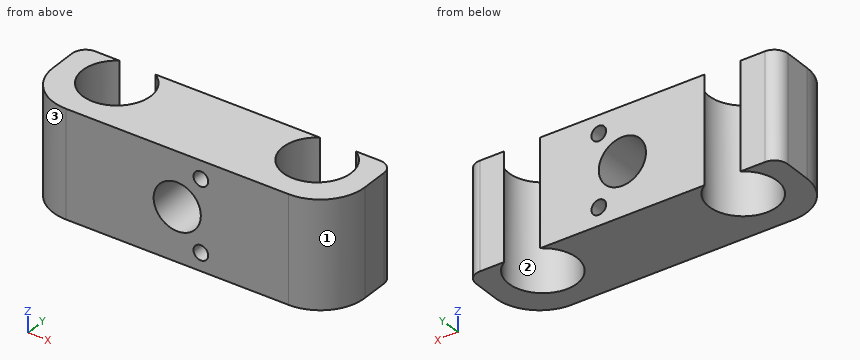
from build123d import *

# Parameters (mm, degrees)
SKETCH_1_W          = 70
SKETCH_1_H          = 19
EXTRUDE_1_DEPTH     = 24
SKETCH_2_R          = 7.65
CUT_EXTRUDE_1_DEPTH = 24
SKETCH_3_R          = 5.3
CUT_EXTRUDE_2_DEPTH = 24
FILLET_1_R          = 10
FILLET_4_R          = 3
FILLET_5_R          = 10
FILLET_6_R          = 3
SKETCH_4_R          = 1.65
CUT_EXTRUDE_3_DEPTH = 24


with BuildPart() as part:
    # 草图1 → 凸台-拉伸1 (new body)
    with BuildSketch(Plane.XY):
        with Locations((35, 9.5)):
            Rectangle(SKETCH_1_W, SKETCH_1_H)
    extrude(amount=EXTRUDE_1_DEPTH)

    # 草图2 → 切除-拉伸1 (cut)
    with BuildSketch(Plane.XY.offset(24)):
        with Locations((57.5, 12.5)):
            Circle(SKETCH_2_R)
        with Locations((12.5, 12.5)):
            Circle(SKETCH_2_R)
    extrude(amount=-CUT_EXTRUDE_1_DEPTH, mode=Mode.SUBTRACT)

    # 草图3 → 切除-拉伸2 (cut)
    with BuildSketch(Plane.XZ):
        with Locations((35, 12)):
            Circle(SKETCH_3_R)
    extrude(amount=-CUT_EXTRUDE_2_DEPTH, mode=Mode.SUBTRACT)

    # 圆角1
    fillet_1_edges = [part.edges().sort_by_distance(p)[0] for p in [
        (0, 0, 12),
    ]]
    fillet(fillet_1_edges, radius=FILLET_1_R)

    # 圆角4
    fillet_4_edges = [part.edges().sort_by_distance(p)[0] for p in [
        (0, 19, 12),
    ]]
    fillet(fillet_4_edges, radius=FILLET_4_R)

    # 圆角5
    fillet_5_edges = [part.edges().sort_by_distance(p)[0] for p in [
        (70, 0, 12),
    ]]
    fillet(fillet_5_edges, radius=FILLET_5_R)

    # 圆角6
    fillet_6_edges = [part.edges().sort_by_distance(p)[0] for p in [
        (70, 19, 12),
    ]]
    fillet(fillet_6_edges, radius=FILLET_6_R)

    # 草图4 → 切除-拉伸3 (cut)
    with BuildSketch(Plane(origin=(0, 19, 0), x_dir=(1, 0, 0), z_dir=(0, 1, 0))):
        with Locations((40.3, -20)):
            Circle(SKETCH_4_R)
        with Locations((40.3, -4)):
            Circle(SKETCH_4_R)
    extrude(amount=-CUT_EXTRUDE_3_DEPTH, mode=Mode.SUBTRACT)


solid = part.part
For this review, take the finished solid that the model builds, in its own axes (mm). Face numbers are marked on the shaded views. Round coordinates to 2 decimals unless told otherwise and drop trailing zeros. Loops run counter-clockwise (first coordinate to the right, second up) from the corner with the lowest first, then second, coordinate; pieces in that order, holes last. Notation, with made-up numbers: (9, 67.25) - (31, 67.25) arc R34 ccw to (31, 102.25) - close; hole circle Ø7 at (29, 5.5). An arc over 180 degrees is marked (long way). Put each result on its own line as item: value. Start each with the question number.
1. Consider section C-C on x = 35. State the section outline as (y, z) points, plus the area to 3 significant figures.
2. Consider section D-D on y = 8.5. State the section outline as (x, z) points, plus the area to 3 significant figures.
3. Consider section B-B on z = 4. State the section outline as (x, y) points, plus the area to 3 significant figures.
4. Mouldability with a two-part tool opening along X and no side actions: class the marked faces 1, 2 and 3 as +X half, -X half, draft (parallel to the pull), parting line (faces both ways), or undercut.
5. Insertion check: P1, Ø2.5, axis at x = 40.3, z = 20, coming from the +Y side; P2, Ø4, axis at y = 7, z = 15.5, coming from the -X side. Each pin has a flat end and moves straight along its axis. Give the tip position at first contact, or say it passes through.
6. Consider section A-A on y = 5.75. State the section outline as (x, z) points.
7. For probe 1 along X at (y, z) = (13.25, 4); probe 2 along X at (y, z) = (12.5, 12.5); probe 3 along Y at (x, z) = (12.5, 8.25), list the stretches that pass through material, from the lowest coordinate up. Write a range as [from, to].
Result sheet:
1. outline: (0, 0) - (19, 0) - (19, 6.7) - (0, 6.7) - close; (0, 17.3) - (19, 17.3) - (19, 24) - (0, 24) - close
1. area: 255 mm^2
2. outline: (0.11, 0) - (5.98, 0) - (5.98, 24) - (0.11, 24) - close; (19.02, 0) - (50.98, 0) - (50.98, 24) - (19.02, 24) - close; (64.02, 0) - (69.89, 0) - (69.89, 24) - (64.02, 24) - close; hole circle Ø10.6 at (35, 12); hole circle Ø3.3 at (40.3, 4); hole circle Ø3.3 at (40.3, 20)
2. area: 943 mm^2
3. outline: (0, 10) arc R10 ccw to (10, 0) - (38.65, 0) - (38.65, 19) - (16.53, 19) arc R7.65 cw (long way) to (8.47, 19) - (3, 19) arc R3 ccw to (0, 16) - close; (41.95, 0) - (60, 0) arc R10 ccw to (70, 10) - (70, 16) arc R3 ccw to (67, 19) - (61.53, 19) arc R7.65 cw (long way) to (53.47, 19) - (41.95, 19) - close
3. area: 865 mm^2
4. face 1: +X half
4. face 2: undercut
4. face 3: -X half
5. P1: through
5. P2: x = 0.05
6. outline: (0.95, 0) - (8.9, 0) - (8.9, 24) - (0.95, 24) - close; (16.1, 0) - (53.9, 0) - (53.9, 24) - (16.1, 24) - close; (61.1, 0) - (69.05, 0) - (69.05, 24) - (61.1, 24) - close; hole circle Ø10.6 at (35, 12); hole circle Ø3.3 at (40.3, 4); hole circle Ø3.3 at (40.3, 20)
7. probe 1: [0, 4.89], [20.11, 38.65], [41.95, 49.89], [65.11, 70]
7. probe 2: [0, 4.85], [20.15, 29.72], [40.28, 49.85], [65.15, 70]
7. probe 3: [0, 4.85]
